Build history of the part. All positions in model axes, mm. Face numbers are marked on the shaded views. A direction names the side the tool comes from. Round coordinates to 2 decimals unless told otherwise and drop trailing zeros. Loops run counter-clockwise (first coordinate to the right, second up) from the corner with the lowest first, then second, coordinate; pieces in that order, holes last. Notation, with made-up numbers: (-13, -8) - (17, -8) arc R16 ccw to (17, 10) - close; hole circle Ø9 at (19, 23.5). An arc over 180 degrees is marked (long way). Put each result on its own line as item: value. Start each with the question number.
from build123d import *

# Parameters (mm, degrees)
F_1_4_28_TAPPED_HOLE1_D = 5.4102
SKETCH4_W               = 25.4
SKETCH4_H               = 25.4
FLATS_DEPTH             = 58.529738397
FILLET1_R               = 1.5875
SKETCH7_R               = 9.525
CUT_EXTRUDE1_DEPTH      = 6.35


with BuildPart() as part:
    # Sketch1 → Revolve1 (revolve)
    with BuildSketch(Plane.XY, mode=Mode.PRIVATE) as revolve1_sk:
        with BuildLine():
            Line((0, 38.1), (-30.48, 38.1))
            Line((-30.48, 38.1), (-30.48, 0))
            Line((-30.48, 0), (-12.7, 0))
            Line((-12.7, 0), (-12.7, 25.4))
            Line((-12.7, 25.4), (-9.525, 25.4))
            ThreePointArc((-9.525, 25.4), (-6.157403955, 24.005096045), (-4.7625, 20.6375))
            Line((-4.7625, 20.6375), (0, 20.6375))
            Line((0, 20.6375), (0, 38.1))
        make_face()
    revolve(revolve1_sk.sketch.rotate(Axis((0, 0, 0), (0, 1, 0)), 180), axis=Axis((0, 0, 0), (0, 1, 0)))

    # 1/4-28 Tapped Hole1 (through all)
    with Locations(Plane(origin=(0, 38.1, 0), x_dir=(1, 0, 0), z_dir=(0, 1, 0))):
        with Locations((0, 0)):
            Hole(F_1_4_28_TAPPED_HOLE1_D / 2)

    # Sketch4 → flats (cut, through all)
    with BuildSketch(Plane(origin=(0, 0, 0), x_dir=(1, 0, 0), z_dir=(0, 1, 0))):
        with Locations((-40.408128771, 0)):
            Rectangle(SKETCH4_W, SKETCH4_H)
        with Locations((40.408128771, 0)):
            Rectangle(SKETCH4_W, SKETCH4_H)
    extrude(amount=FLATS_DEPTH, mode=Mode.SUBTRACT)

    # Sketch6 → 3/8 NPT Tapped Hole1 (revolve, cut)
    with BuildSketch(Plane(origin=(27.708128771, 15.875, 0), x_dir=(0, 0, -1), z_dir=(0, 1, 0))):
        Polygon((0, 0), (0, 21.814582582), (7.1374, 17.526), (7.1374, 10.414), (8.263205494, 10.414), (8.5750146, 0), align=None)
    f_3_8_npt_tapped_hole1 = revolve(axis=Axis((34.058128771, 15.875, 0), (-1, 0, 0)), mode=Mode.SUBTRACT)

    # Mirror1: 3/8 NPT Tapped Hole1 across plane
    add(f_3_8_npt_tapped_hole1.mirror(Plane(origin=(0, 0, 0), x_dir=(0, 0, 1), z_dir=(1, 0, 0))), mode=Mode.SUBTRACT)

    # Fillet1
    fillet1_edges = [part.edges().sort_by_distance(p)[0] for p in [
        (-12.7, 25.4, 0),
    ]]
    fillet(fillet1_edges, radius=FILLET1_R)

    # Sketch7 → Cut-Extrude1 (cut)
    with BuildSketch(Plane(origin=(0, 38.1, 0), x_dir=(1, 0, 0), z_dir=(0, 1, 0))):
        with Locations(Location((0, 0, 0), (0, 0, 180))):
            Circle(SKETCH7_R)
    extrude(amount=-CUT_EXTRUDE1_DEPTH, mode=Mode.SUBTRACT)


solid = part.part
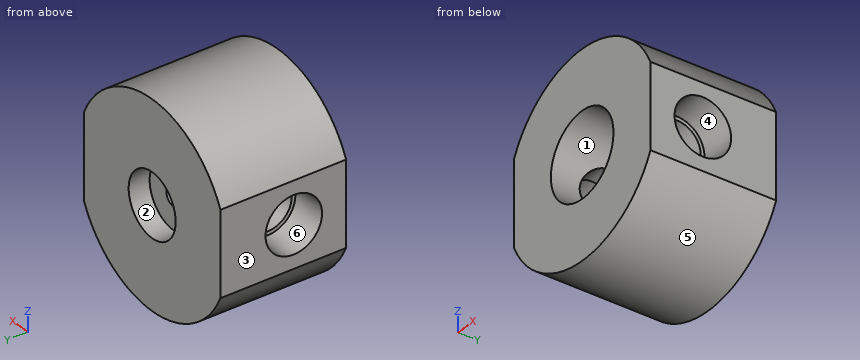
1) Slice it at D-D, the plane z = 0. State how many separate pieces and enclosed holes the cut face has, and give its area (3 significant figures).
2) Slice it at B-B, the plane y = 27. Write the cut outline in (x, z).
3) Pull direction X, two halves, no side cores. Call the marked faces 1, 2, 3 and 4: pulls with the +X half, pulls with the -X half, needs draft (parallel to the pull), parting line crosses it, or undercut.
4) Drop flat-ended pins along their axis: pin 1 Ø4 at (y, z) = (12.5, -2.5) entering from +X; pin 2 Ø5 at (x, z) = (0.5, -0.5) entering from -Y; pin 3 Ø6 at (x, y) = (8, 11.5) entering from +Z; pin 4 Ø6 at (x, y) = (20.5, 25.5) entering from +Z. Give the stop position or say it passes through.
5) Slice it at C-C, the plane x = 15. Write the cut outline in (y, z) (3 decimals).
6) Which spindle directions (+Z, -Z, +X, -X, +Y, -Y) get a long thin tool onto all of the face, cutting with end or side? Do the marked faces 5 and 6. Say none if no direction does.
7) Drill centre lines: line 1 (Z direction, x = 0, y = 28.25); line 2 (Z direction, x = 0, y = 35) (3 decimals); line 3 (Y direction, x = -14, z = 0). Where is each one in solid material? Low to high. Write a range as [from, to].
Taken from the geometry:
1. separate pieces: 4
1. enclosed holes: 0
1. area: 859 mm2
2. outline: (-27.71, -12.7) arc R30.48 ccw to (27.71, -12.7) - (27.71, 12.7) arc R30.48 ccw to (-27.71, 12.7) - close; hole circle Ø5.41 at (0, 0)
3. face 1: undercut
3. face 2: undercut
3. face 3: pulls with the -X half
3. face 4: pulls with the +X half
4. pin 1: passes through
4. pin 2: stops at y = 20.64
4. pin 3: stops at z = 30.07
4. pin 4: stops at z = 24.96
5. outline: (0, -26.534) - (38.1, -26.534) - (38.1, 26.534) - (0, 26.534) - close; hole circle Ø14.275 at (15.875, 0)
6. face 5: -Z, +Y, -Y
6. face 6: -X
7. line 1: z = [-30.48, -2.71], [2.71, 30.48]
7. line 2: z = [-30.48, -9.525], [9.525, 30.48]
7. line 3: y = [0, 8.74], [23.01, 38.1]
